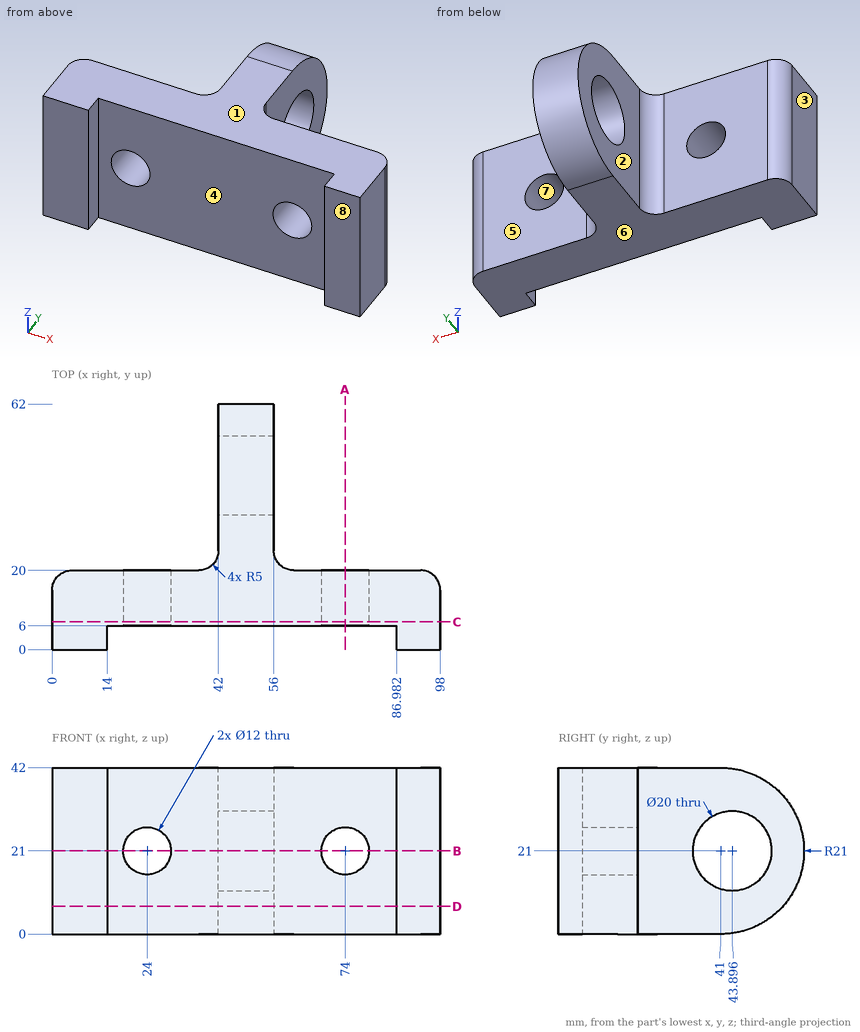
The drawing under review shows one solid part. Ordinate dimensions are in mm from its lowest x, y, z. A direction names the side the tool comes from. Give positions to 0.01 mm unless a question says otherwise; leave off trailing zeros. Order: outer loops, then holes, each group sorted by start corner. A loop starts at its lowest first (then second) coordinate and runs counter-clockwise, first axis right, second up. Notation, with made-up numbers: (46, 24) - (58, 24) arc R22 cw to (58, 52) - close; hole circle Ø7 at (-38.5, 48). An arc over 180 degrees is marked (long way). Answer as a JSON object with one key per item and string values. Group by question number.
Item 1: Take a section at A-A on x = 74. Give the boundary of the cut face in (y, z).
Item 2: Take a section at D-D on z = 7. Give the boundary of the cut face in (x, y).
Item 3: Draft analysis for pull direction Z (two halves, no side actions). For the marked faces 6, 7 and 8, state which applies: pulls with the +Z half, pulls with the -Z half, needs draft (parallel to the pull), parting line crosses it, or undercut.
Item 4: Take a section at B-B on z = 21. Give the boundary of the cut face in (x, y) (1 decimal), and give its area (3 significant figures).
Item 5: Wall thickness on line 1 along X through (y, z) = (13.5, 21); line 2 along Y through (x, z) = (46.5, 21) (1 decimal); line 3 along X through (y, z) = (8.5, 19.5): over which ranges is each line inside the solid? List them lowest first.
Item 6: Take a section at C-C on y = 7. Give the boundary of the cut face in (x, z).
Item 7: Machinability: for the marked faces 1, 2, 3, 4 and 5, which of the approach directions +Z, -Z, +X, -X, +Y, -Y give a long, thin tool a straight path to every point of the face, cutting with its end or side? Answer none if there is none.
Item 8: Clearance check with flat-ended pins moving along their axes: pin 1 Ø1.5 at (x, z) = (59, 18) entering from -Y; pin 2 Ø9.5 at (x, z) = (80, 24.5) entering from +Y; pin 3 Ø2 at (x, z) = (37, 7.5) entering from +Y; pin 4 Ø9.5 at (x, z) = (74, 21) entering from -Y. State where each tip first meets the part, or that it passes through.
Reported:
{
 "1": {"outline": "(6, 0) - (20, 0) - (20, 15) - (6, 15) - close; (6, 27) - (20, 27) - (20, 42) - (6, 42) - close"},
 "2": {"outline": "(0, 0) - (14, 0) - (14, 6) - (86.98, 6) - (86.98, 0) - (98, 0) - (98, 15) arc R5 ccw to (93, 20) - (61, 20) arc R5 cw to (56, 25) - (56, 56.65) - (42, 56.65) - (42, 25) arc R5 cw to (37, 20) - (5, 20) arc R5 ccw to (0, 15) - close"},
 "3": {"face 6": "pulls with the -Z half", "face 7": "undercut", "face 8": "needs draft"},
 "4": {"outline": "(0, 0) - (14, 0) - (14, 6) - (18, 6) - (18, 20) - (5, 20) arc R5 ccw to (0, 15) - close; (30, 6) - (68, 6) - (68, 20) - (61, 20) arc R5 cw to (56, 25) - (56, 33.9) - (42, 33.9) - (42, 25) arc R5 cw to (37, 20) - (30, 20) - close; (42, 53.9) - (56, 53.9) - (56, 62) - (42, 62) - close; (80, 6) - (87, 6) - (87, 0) - (98, 0) - (98, 15) arc R5 ccw to (93, 20) - (80, 20) - close", "area": "1,490 mm^2"},
 "5": {"line 1": "0 to 18, 30 to 68, 80 to 98", "line 2": "6 to 33.9, 53.9 to 62", "line 3": "0 to 18.19, 29.81 to 68.19, 79.81 to 98"},
 "6": {"outline": "(0, 0) - (98, 0) - (98, 42) - (0, 42) - close; hole circle Ø12 at (24, 21); hole circle Ø12 at (74, 21)"},
 "7": {"face 1": "+Z, +X, -X, +Y, -Y", "face 2": "+Z, -Z, -X, +Y", "face 3": "+Z, -Z, -X, +Y, -Y", "face 4": "+Z, -Z, -Y", "face 5": "+Z, -Z, +X, +Y"},
 "8": {"pin 1": "y = 6", "pin 2": "y = 20", "pin 3": "y = 20.1", "pin 4": "through"}
}
